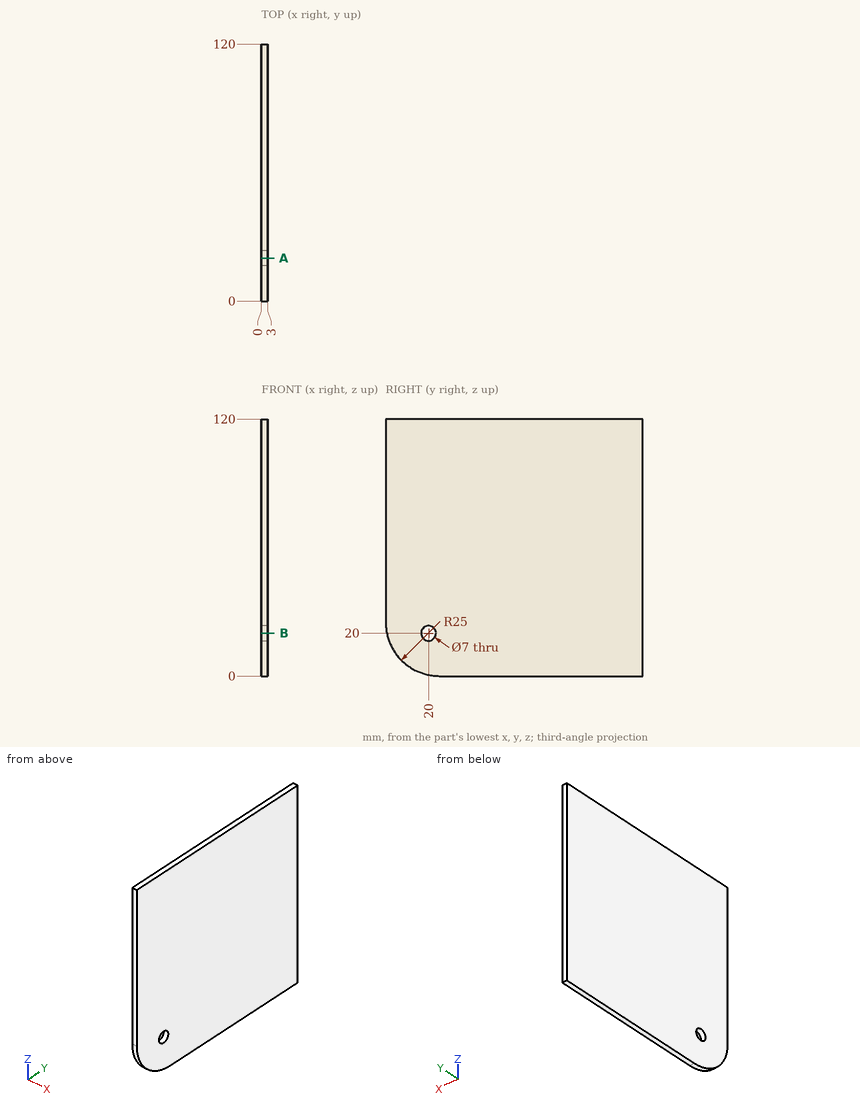
Input: dimensioned drawing with shaded views. Units: mm. Origin: part minimum x, y, z. Round coordinates to 2 decimals unless told otherwise and drop trailing zeros. Order: outer loops, then holes, each group sorted by start corner. A loop starts at its lowest first (then second) coordinate and runs counter-clockwise, first axis right, second up. Notation, with made-up numbers: (-22.5, -11.75) -> (19.5, -11.75) arc R30 cw to (19.5, 15.25) -> close; hole circle Ø6 at (66.25, 57). An arc over 180 degrees is marked (long way). Put each result on its own line as item: value. Start each with the question number.
Q1. Line query: probe 1 along Z at (x, y) = (1.65, 21.5); probe 2 along Y at (x, z) = (1.7, 20); probe 3 along Y at (x, z) = (0.5, 17). Output: solid intervals per line, ascending.
Q2. Section A-A on y = 20. Return the cut outline in (x, z), and give its area (3 significant figures).
Ans:
1. probe 1: z = 0.25 to 16.84, 23.16 to 120
1. probe 2: y = 0.51 to 16.5, 23.5 to 120
1. probe 3: y = 1.31 to 18.2, 21.8 to 120
2. outline: (0, 0.51) -> (3, 0.51) -> (3, 16.5) -> (0, 16.5) -> close; (0, 23.5) -> (3, 23.5) -> (3, 120) -> (0, 120) -> close
2. area: 337 mm2
